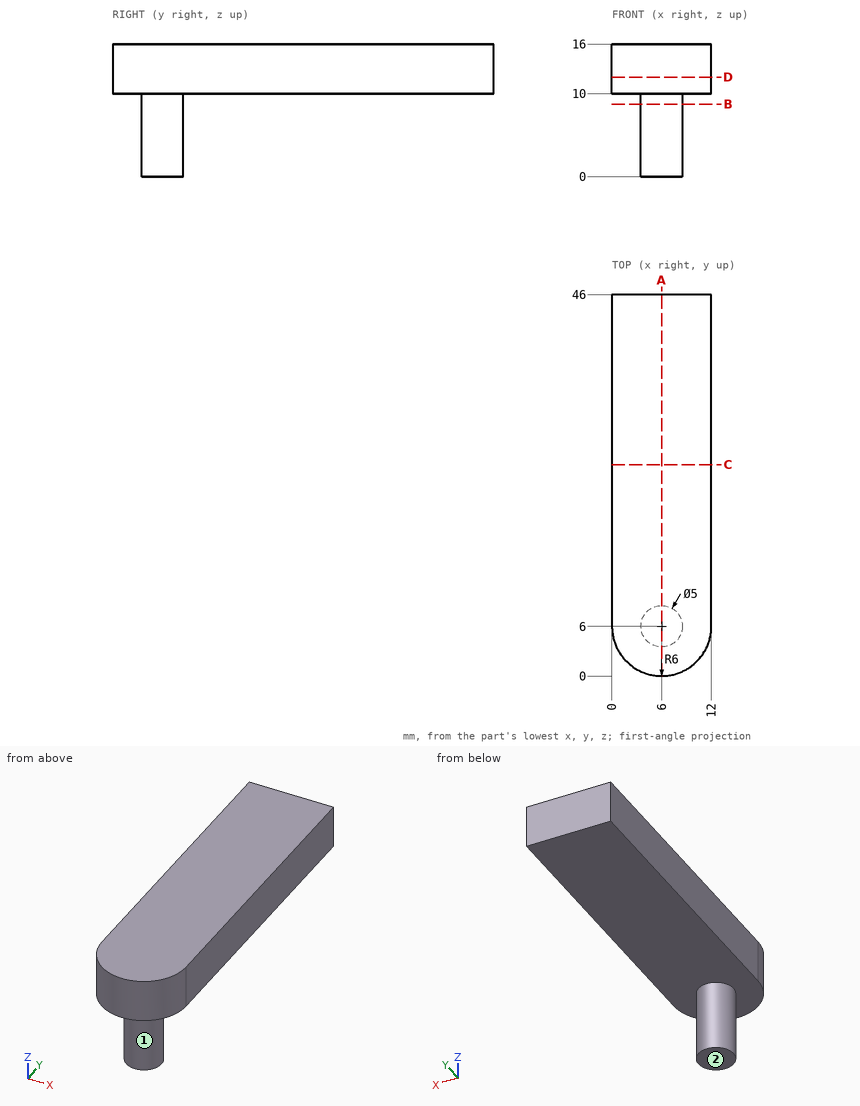
Answer from the drawing. Dimensions are ordinates in mm from the lowest x, y and z of the part. A direction names the side the tool comes from. Give positions to 0.01 mm unless a question says otherwise; leave off trailing zeros. Loops run counter-clockwise (first coordinate to the right, second up) from the corner with the lowest first, then second, coordinate; pieces in that order, holes last. Notation, with made-up numbers: (72.25, 68.25) -> (117.25, 68.25) arc R33 ccw to (117.25, 98.25) -> close; hole circle Ø8 at (82.25, 5). An arc over 180 degrees is marked (long way). One line per question, with ' | ' between items. Start each with the question number.
1) Straight lines are drawn through the part: L1, parallel to Z at x = 1.25, y = 10; L2, parallel to Y at x = 3.75, z = 11.25; L3, parallel to Y at x = 6.5, z = 14.5. For each, find the intervals that lie inside material, in ascending order.
2) Section B-B, the plane z = 8.75 is taken. Determine the outline of the cut face in (x, y), then the cut area to 3 significant figures.
3) Section D-D, the plane z = 12 is taken. Determine the outline of the cut face in (x, y).
4) For the marked faces 1 and 2, determine the directions among +Z, -Z, +X, -X, +Y, -Y from which every point of the face is accessible in a straight line to the end or side of a thin tool.
5) Section C-C, the plane y = 25.5 is taken. Determine the outline of the cut face in (x, z), then the cut area to 3 significant figures.
6) Each of these flat-tipped pins is pushed along its axis until it touches: pin 1 (5 mm diameter, centred on x = 4, z = 5, fed in from -Y); pin 2 (3 mm diameter, centred on x = 6.5, z = 4.5, fed in from +Y); pin 3 (1.5 mm diameter, centred on x = 3.5, z = 5, fed in from -Y). Where does it stop, or does it pass through?
7) Section A-A, the plane x = 6 is taken. Determine the outline of the cut face in (y, z).
Resolved:
1) L1: 10 to 16 | L2: 0.44 to 46 | L3: 0.02 to 46
2) outline: circle Ø5 at (6, 6) | area: 19.6 mm2
3) outline: (0, 6) arc R6 ccw to (12, 6) -> (12, 46) -> (0, 46) -> close
4) face 1: -Z | face 2: -Z, +X, -X, +Y, -Y
5) outline: (0, 10) -> (12, 10) -> (12, 16) -> (0, 16) -> close | area: 72.0 mm2
6) pin 1: y = 3.5 | pin 2: y = 8.5 | pin 3: y = 4.21
7) outline: (0, 10) -> (3.5, 10) -> (3.5, 0) -> (8.5, 0) -> (8.5, 10) -> (46, 10) -> (46, 16) -> (0, 16) -> close
